Input: part model. Units: mm. Frame: model coordinates. A direction names the side the tool comes from. Round coordinates to 2 decimals unless told otherwise and drop trailing zeros. Order: outer loops, then holes, each group sorted by start corner. A loop starts at its lowest first (then second) coordinate and runs counter-clockwise, first axis right, second up.
Item 1: Mould query, pull axis Y, two halves, no side actions, for faces 3 (the flat face through (-2, 18.057, 1)), 4 (the flat face through (6.088, 3, 1)), 5 (the flat face through (-2, 17.057, 2)). Classes: released by +Y, released by -Y, zero draft, split by the parting line, or undercut.
Item 2: Cut plane A-A on z = 2. Output: boundary loops of the cut face in (x, y), then the cut area to 3 significant figures.
Item 3: First-contact query: pin 1 (6 mm diameter, centred on x = -7.5, y = 3.5, fed in from +Z); pin 2 (4 mm diameter, centred on x = 0, y = -2.5, fed in from +Z). Flat tips, straight axial feed; report the tip coordinate or a pass-through.
Item 4: Reachability of faces 1 (the flat face through (-8.412, 3, 2)), 2 (the flat face through (-2, 3, 0)) from +Z, -Z, +X, -X, +Y, -Y: full face, straight path, thin tool, end or side. Return the list, or none.
Item 5: Cut plane C-C on y = 12. Output: boundary loops of the cut face in (x, z).
Item 6: Line query: L1, parallel to X at y = -5.5, z = 2.3; L2, parallel to Y at x = -7, z = 2.1; L3, parallel to Z at x = -5, y = 9.5. Output: solid intervals per line, ascending.
Item 7: Cut plane B-B on x = 3.25. Output: boundary loops of the cut face in (y, z), then the cut area to 3 significant figures.
```python
from build123d import *

# Parameters (mm, degrees)
F0_W     = 15.5
F0_H     = 30.5
F0_W_2   = 13.5
F0_H_2   = 28.5
F1_DEPTH = 3
F2_DEPTH = 1.5
F3_R     = 0.5


with BuildPart() as f1:
    # F0 (on Top) → F1 (new body)
    with BuildSketch(Plane.XY):
        with Locations((-1.661532, 2.806597)):
            Rectangle(F0_W, F0_H)
        with Locations((-1.661532, 2.806597)):
            Rectangle(F0_W_2, F0_H_2, mode=Mode.SUBTRACT)
    extrude(amount=F1_DEPTH)

    # F0 (on Top) → F2 (join)
    with BuildSketch(Plane.XY):
        with Locations((-1.661532, 2.806597)):
            Rectangle(F0_W_2, F0_H_2)
    extrude(amount=F2_DEPTH)

    # F3
    f3_edges = [f1.edges().sort_by_distance(p)[0] for p in [
        (6.088468, -12.443403, 1.5),
        (6.088468, 18.056597, 1.5),
        (6.088468, 2.806597, 0),
        (6.088468, 2.806597, 3),
        (-9.411532, -12.443403, 1.5),
        (-1.661532, -12.443403, 0),
        (-1.661532, -12.443403, 3),
        (-9.411532, 18.056597, 1.5),
        (-9.411532, 2.806597, 0),
        (-9.411532, 2.806597, 3),
        (-1.661532, 18.056597, 0),
        (-1.661532, 18.056597, 3),
    ]]
    fillet(f3_edges, radius=F3_R)


solid = f1.part
```
From the geometry:
1. face 3: released by +Y
1. face 4: zero draft
1. face 5: undercut
2. outline: (-9.41, -11.94) arc R0.5 ccw to (-8.91, -12.44) - (5.59, -12.44) arc R0.5 ccw to (6.09, -11.94) - (6.09, 17.56) arc R0.5 ccw to (5.59, 18.06) - (-8.91, 18.06) arc R0.5 ccw to (-9.41, 17.56) - close; hole (-8.41, -11.44) - (5.09, -11.44) - (5.09, 17.06) - (-8.41, 17.06) - close
2. area: 87.8 mm2
3. pin 1: stops at z = 3
3. pin 2: stops at z = 1.5
4. face 1: +Z
4. face 2: -Z, +X, -X, +Y, -Y
5. outline: (-9.41, 0.5) arc R0.5 ccw to (-8.91, 0) - (5.59, 0) arc R0.5 ccw to (6.09, 0.5) - (6.09, 2.5) arc R0.5 ccw to (5.59, 3) - (5.09, 3) - (5.09, 1.5) - (-8.41, 1.5) - (-8.41, 3) - (-8.91, 3) arc R0.5 ccw to (-9.41, 2.5) - close
6. L1: x = -9.41 to -8.41, 5.09 to 6.09
6. L2: y = -12.44 to -11.44, 17.06 to 18.06
6. L3: z = 0 to 1.5
7. outline: (-12.44, 0.5) arc R0.5 ccw to (-11.94, 0) - (17.56, 0) arc R0.5 ccw to (18.06, 0.5) - (18.06, 2.5) arc R0.5 ccw to (17.56, 3) - (17.06, 3) - (17.06, 1.5) - (-11.44, 1.5) - (-11.44, 3) - (-11.94, 3) arc R0.5 ccw to (-12.44, 2.5) - close
7. area: 48.5 mm2
